Geometry check sheet. Reference: the model listing, model coordinates, mm. A direction names the side the tool comes from. Give positions to 0.01 mm unless a question says otherwise; leave off trailing zeros. Write each loop counter-clockwise with the first axis right and the second up, starting at its lowest first coordinate (ties: lowest second). Pieces come first, ordered by that corner, then holes. Notation, with made-up numbers: (54, 26) - (79, 26) arc R27 ccw to (79, 44) - close; hole circle Ø2 at (52.25, -2). An arc over 180 degrees is marked (long way). Use a Markdown table: item, result.
```python
from build123d import *

# Parameters (mm, degrees)
SKETCH1_W                    = 58.25
SKETCH1_H                    = 68.58
BOSS_EXTRUDE1_DEPTH          = 6.575
FILLET1_R                    = 6
BOSS_EXTRUDE2_DEPTH          = 3.175
SKETCH6_W                    = 17.78
SKETCH6_H                    = 5.08
BOSS_EXTRUDE3_DEPTH          = 3.81
F_30_0_1285_DIAMETER_HOLE1_D = 3.2639
FILLET2_R                    = 2
CUT_EXTRUDE1_DEPTH           = 55.710248126


with BuildPart() as part:
    # Sketch1 → Boss-Extrude1 (new, symmetric)
    with BuildSketch(Plane.XY):
        Rectangle(SKETCH1_W, SKETCH1_H)
    extrude(amount=BOSS_EXTRUDE1_DEPTH, both=True)

    # Fillet1
    fillet1_edges = [part.edges().sort_by_distance(p)[0] for p in [
        (29.125, -34.29, 0),
        (-29.125, -34.29, 0),
        (-29.125, 34.29, 0),
        (29.125, 34.29, 0),
    ]]
    fillet(fillet1_edges, radius=FILLET1_R)

    # Sketch2 → Boss-Extrude2 (add)
    with BuildSketch(Plane(origin=(0, 0, -6.575), x_dir=(-1, 0, 0), z_dir=(0, 0, -1))):
        Polygon((-29.125, 14.29), (-37.975, 8.65), (-37.975, -8.65), (-29.125, -14.29), align=None)
    boss_extrude2 = extrude(amount=-BOSS_EXTRUDE2_DEPTH)

    # Sketch6 → Boss-Extrude3 (add)
    with BuildSketch(Plane.XZ.offset(34.29)):
        with Locations((-12.615, 2.54)):
            Rectangle(SKETCH6_W, SKETCH6_H)
    boss_extrude3 = extrude(amount=BOSS_EXTRUDE3_DEPTH)

    # #30 (0.1285) Diameter Hole1 (through all)
    with Locations(Plane.XY.offset(-3.4)):
        with Locations((34.29, 0), (34.29, -5.588)):
            f_30_0_1285_diameter_hole1 = Hole(F_30_0_1285_DIAMETER_HOLE1_D / 2)

    # Mirror1: Boss-Extrude2, Boss-Extrude3, #30 (0.1285) Diameter Hole1 across plane
    add(boss_extrude2.mirror(Plane(origin=(0, 0, 0), x_dir=(0, 0, 1), z_dir=(1, 0, 0))))
    add(boss_extrude3.mirror(Plane(origin=(0, 0, 0), x_dir=(0, 0, 1), z_dir=(1, 0, 0))))
    add(f_30_0_1285_diameter_hole1.mirror(Plane(origin=(0, 0, 0), x_dir=(0, 0, 1), z_dir=(1, 0, 0))), mode=Mode.SUBTRACT)

    # Fillet2
    fillet2_edges = [part.edges().sort_by_distance(p)[0] for p in [
        (29.125, 14.29, -4.9875),
        (29.125, -14.29, -4.9875),
        (37.975, -8.65, -4.9875),
        (37.975, 8.65, -4.9875),
        (-29.125, -14.29, -4.9875),
        (-29.125, 14.29, -4.9875),
        (-37.975, 8.65, -4.9875),
        (-37.975, -8.65, -4.9875),
    ]]
    fillet(fillet2_edges, radius=FILLET2_R)

    # Sketch5 → Cut-Extrude1 (cut, through all)
    with BuildSketch(Plane.XY.offset(-3.4)):
        with BuildLine():
            Line((-33.6169, -7.20725), (-34.9631, -7.20725))
            ThreePointArc((-34.9631, -7.20725), (-36.58235, -5.588), (-34.9631, -3.96875))
            Line((-34.9631, -3.96875), (-33.6169, -3.96875))
            ThreePointArc((-33.6169, -3.96875), (-31.99765, -5.588), (-33.6169, -7.20725))
        make_face()
    extrude(amount=-CUT_EXTRUDE1_DEPTH, mode=Mode.SUBTRACT)


solid = part.part
```
1) Set-up check for faces 1 (the flat face through (-21.505, -36, 3)), 2 (the flat face through (3.725, -36, 3)), 3 (the flat face through (13, -36, 0)), 4 (the flat face through (-32, 0, -3.4)), 5 (the cylindrical face through (-32, -5.55, -4.97)): record each of +Z, -Z, +X, -X, +Y, -Y from which the full face is reachable in a straight line by a thin tool's end or side.
Working result:
| item | result |
|---|---|
| face 1 | +Z, -Z, -X, -Y |
| face 2 | +Z, -Z, -Y |
| face 3 | -Z, +X, -X, -Y |
| face 4 | +Z, -X, +Y, -Y |
| face 5 | +Z, -Z |
2) Section check A-A on y = 0. Record the boundary of the cut face in (x, z) (3 decimals).
Working result:
| item | result |
|---|---|
| outline | (-37.975, -6.575) - (-35.922, -6.575) - (-35.922, -3.4) - (-37.975, -3.4) - close; (-32.658, -6.575) - (32.658, -6.575) - (32.658, -3.4) - (29.125, -3.4) - (29.125, 6.575) - (-29.125, 6.575) - (-29.125, -3.4) - (-32.658, -3.4) - close; (35.922, -6.575) - (37.975, -6.575) - (37.975, -3.4) - (35.922, -3.4) - close |
3) Section check B-B on x = 34.29. Record the boundary of the cut face in (y, z) (3 decimals), then the cut area to 3 significant figures.
Working result:
| item | result |
|---|---|
| outline | (-10.998, -6.575) - (-7.22, -6.575) - (-7.22, -3.4) - (-10.998, -3.4) - close; (-3.956, -6.575) - (-1.632, -6.575) - (-1.632, -3.4) - (-3.956, -3.4) - close; (1.632, -6.575) - (10.998, -6.575) - (10.998, -3.4) - (1.632, -3.4) - close |
| area | 49.1 mm² |
4) Depth check by flat-ended pin: P1, Ø4.5, axis at x = -35.5, y = -3, coming from the +Z side; P2, Ø1.9, axis at x = 16, y = -37, coming from the -Z side; P3, Ø6, axis at y = 23.5, z = -3, coming from the +X side (3 decimals); P4, Ø5, axis at x = -34.29, y = 0, coming from the -Z side (3 decimals). Enter the tip coordinate at first touch or a pass-through.
Working result:
| item | result |
|---|---|
| P1 | stops at z = -3.4 |
| P2 | stops at z = 0 |
| P3 | stops at x = 29.125 |
| P4 | stops at z = -6.575 |
5) Mould release check, pull along Y, two halves, no side actions. Record for faces 6 (the flat face through (32, 0, -3.4)), 7 (the cylindrical face through (-33, -1, -5)), 8 (the cylindrical face through (32.733, 0.49, -5.01)), 9 (the cylindrical face through (37.72, -8.53, -4.97)): pulls with the +Y half, pulls with the -Y half, needs draft (parallel to the pull), parting line crosses it, or undercut.
Working result:
| item | result |
|---|---|
| face 6 | needs draft |
| face 7 | undercut |
| face 8 | undercut |
| face 9 | pulls with the -Y half |
6) Section check C-C on z = -4.5. Count the separate pieces of the cut face and the enclosed holes in it, then the cut area to 3 significant figures.
Working result:
| item | result |
|---|---|
| separate pieces | 1 |
| enclosed holes | 4 |
| area | 4,330 mm² |
7) Section check D-D on y = 11. Record the boundary of the cut face in (x, z) (1 decimal).
Working result:
| item | result |
|---|---|
| outline | (-34.3, -6.6) - (34.3, -6.6) - (34.3, -3.4) - (29.1, -3.4) - (29.1, 6.6) - (-29.1, 6.6) - (-29.1, -3.4) - (-34.3, -3.4) - close |
8) Material ranges on L1, parallel to Y at x = -34.29, z = -4.8; L2, parallel to X at y = -17.5, z = 5 (3 decimals); L3, parallel to Y at x = 33, z = -5.5, recorded low to high. Write a range as from..to.
Working result:
| item | result |
|---|---|
| L1 | y = -11..-7.22, -3.96..-1.63, 1.63..11 |
| L2 | x = -29.125..29.125 |
| L3 | y = -11.82..-6.59, -4.59..-1, 1..11.82 |
